Geometry: see drawing. Coordinates: mm, zero at the bounding-box minimum. A direction names the side the tool comes from. Give positions to 0.01 mm unless a question says otherwise; leave off trailing zeros. Loops run counter-clockwise (first coordinate to the right, second up) from the corner with the lowest first, then second, coordinate; pieces in that order, holes last. Notation, with made-up numbers: M -28.75,41 L -7.75,41 A14 cw -7.75,45 Z; hole C 25,31 d10. An arc over 180 degrees is marked long. Answer in a Markdown table with one row per item.
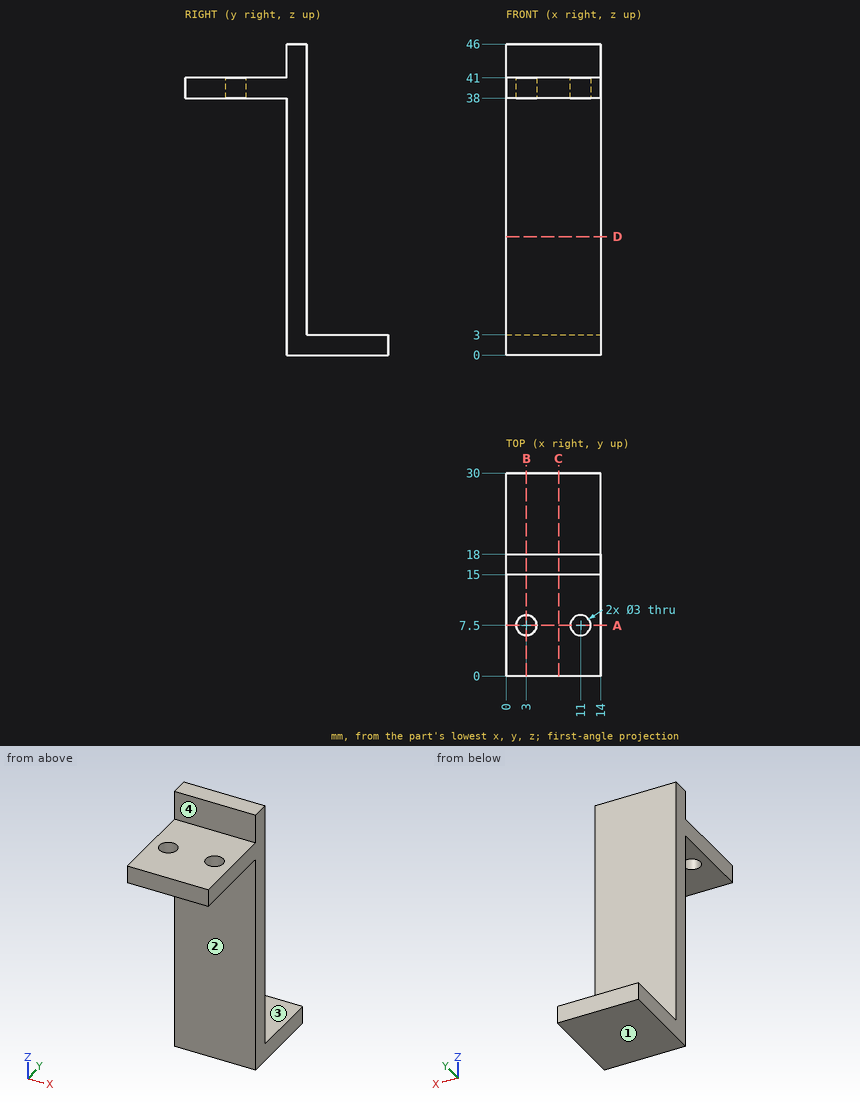
1) Section D-D, the plane z = 17.5. Return loops of the section in (x, y), then the cut area to 3 significant figures.
Reply:
| item | result |
|---|---|
| outline | M 0,15 L 14,15 L 14,18 L 0,18 Z |
| area | 42.0 mm² |
2) Material intervals for L1, parallel to Y at x = 3, z = 39; L2, parallel to Z at x = 4.5, y = 20.5; L3, parallel to Y at x = 2.5, z = 15, sorted ascending.
Reply:
| item | result |
|---|---|
| L1 | y = 0 to 6, 9 to 18 |
| L2 | z = 0 to 3 |
| L3 | y = 15 to 18 |
3) Section C-C, the plane x = 7.75. Return loops of the section in (y, z), then the cut area to 3 significant figures.
Reply:
| item | result |
|---|---|
| outline | M 0,38 L 15,38 L 15,0 L 30,0 L 30,3 L 18,3 L 18,46 L 15,46 L 15,41 L 0,41 Z |
| area | 219 mm² |
4) Section A-A, the plane y = 7.5. Return loops of the section in (x, z).
Reply:
| item | result |
|---|---|
| outline | M 0,38 L 1.5,38 L 1.5,41 L 0,41 Z; M 4.5,38 L 9.5,38 L 9.5,41 L 4.5,41 Z; M 12.5,38 L 14,38 L 14,41 L 12.5,41 Z |
5) Pin query (flat end, axial travel): pin 1 Ø2 at (x, y) = (8.5, 12.5) entering from +Z; pin 2 Ø7 at (x, z) = (9.5, 15.5) entering from -Y; pin 3 Ø7 at (x, y) = (5, 7) entering from -Z. Return the tip coordinate at first contact, or that it passes through.
Reply:
| item | result |
|---|---|
| pin 1 | stops at z = 41 |
| pin 2 | stops at y = 15 |
| pin 3 | stops at z = 38 |
6) Section B-B, the plane x = 3. Return loops of the section in (y, z).
Reply:
| item | result |
|---|---|
| outline | M 0,38 L 6,38 L 6,41 L 0,41 Z; M 9,38 L 15,38 L 15,0 L 30,0 L 30,3 L 18,3 L 18,46 L 15,46 L 15,41 L 9,41 Z |
7) Set-up query: the marked faces 1, 2, 3 and 4. Return all of +Z, -Z, +X, -X, +Y, -Y with unobstructed straight access to the full face (end or side cutting, diameter ignored); none if empty.
Reply:
| item | result |
|---|---|
| face 1 | -Z, +X, -X, +Y, -Y |
| face 2 | -Z, +X, -X, -Y |
| face 3 | +Z, +X, -X, +Y |
| face 4 | +Z, +X, -X, -Y |
